Here's how the part is built. I have some questions about the finished solid (model axes, mm). A direction names the side the tool comes from. Give positions to 0.01 mm unless a question says otherwise; leave off trailing zeros. Order: outer loops, then holes, each group sorted by start corner. A loop starts at its lowest first (then second) coordinate and runs counter-clockwise, first axis right, second up. Notation, with made-up numbers: (73, 72) -> (106, 72) arc R21 cw to (106, 87) -> close; hole circle Ø6 at (-5, 22.25). An arc over 180 degrees is marked (long way). Write each question's results on one line, items separated by ' | '. Start each with the question number.
Q1. Imagine slicing it at B-B, the plane z = -34. State how many separate pieces and enclosed holes the cut face has, then the cut area to 3 significant figures.
Q2. I need wall thicknesses on line 1 along X through (y, z) = (13, -24); line 2 along Z through (x, y) = (69, 6.75); line 3 along Z through (x, y) = (31, 14). Which ranges of each line are inside material? Lowest first, please. Write a range as [from, to].
Q3. Thinking about a two-plate mould opening in Y: for faces 1 (the face through (95.504, 13, -17)), 2 (the face through (22, 25.375, -19)), 3 (the face through (81.08, 12.74, -14.7)), which applies, pulls with the +Y half, pulls with the -Y half, needs draft (parallel to the pull), parting line crosses it, or undercut?
Q4. I'm going to push flat-ended pins straight in: pin 1 (4 mm diameter, centred on x = 49.784, z = 0, fed in from -Y); pin 2 (13 mm diameter, centred on x = 69.85, y = 12.7, fed in from -Z); pin 3 (1 mm diameter, centred on x = 20.5, z = -9, fed in from -Y); pin 4 (1 mm diameter, centred on x = 16.5, y = 7.5, fed in from +Z). Where does each tip first touch, or does it pass through?
Q5. Imagine slicing it at C-C, the plane y = 2.5. Please give me the cut outline in (x, z), then the cut area to 3 significant figures.
Q6. For faces 4 (the face through (70, 0, -17)), 5 (the face through (75.156, 14.371, -25.858)), 6 (the face through (65.25, 14.37, -8.33)), which set-ups out of +Z, -Z, +X, -X, +Y, -Y let a thin tool reach every point of the face, with its end or its side?
```python
from build123d import *

# Parameters (mm, degrees)
BOSS_EXTRUDE1_DEPTH = 25.4
SKETCH2_W           = 44.704
SKETCH2_H           = 0.0254
CUT_EXTRUDE1_DEPTH  = 107.377492525
SKETCH3_R           = 2.286
CUT_EXTRUDE2_DEPTH  = 107.377492525


# Read off the part's stored shape, not the designer's step: 1/4 NPT Tapped Hole1
with BuildPart() as part:
    # Sketch1 → Boss-Extrude1 (new body)
    with BuildSketch(Plane(origin=(0, 0, 0), x_dir=(1, 0, 0), z_dir=(0, 1, 0))):
        Polygon((44.704, -5.08), (95.504, -5.08), (95.504, 39.37), (0, 39.37), (0, 0), (44.704, 0), align=None)
    extrude(amount=BOSS_EXTRUDE1_DEPTH)

    # Sketch2 → Cut-Extrude1 (cut, through all)
    with BuildSketch(Plane.XY):
        with Locations((22.352, 25.3873)):
            Rectangle(SKETCH2_W, SKETCH2_H)
        with Locations((22.352, 0.0127)):
            Rectangle(SKETCH2_W, SKETCH2_H)
    extrude(amount=-CUT_EXTRUDE1_DEPTH, mode=Mode.SUBTRACT)

    # Sketch3 → Cut-Extrude2 (cut, through all)
    with BuildSketch(Plane(origin=(0, 25.4, 0), x_dir=(1, 0, 0), z_dir=(0, 1, 0))):
        with Locations(Location((49.784, 0, 0), (0, 0, 270))):
            Circle(SKETCH3_R)
        with Locations(Location((84.328, 34.544, 0), (0, 0, 270))):
            Circle(SKETCH3_R)
    extrude(amount=-CUT_EXTRUDE2_DEPTH, mode=Mode.SUBTRACT)

    # 1/4 NPT Tapped Hole1 outline → 1/4 NPT Tapped Hole1 (revolve, cut)
    with BuildSketch(Plane(origin=(69.85, 12.7, 0), x_dir=(1, 0, 0), z_dir=(0, -1, 0))):
        Polygon((5.5626, -22.352), (0, -19.009652721), (0, -39.37), (6.8545837, -39.37), (6.557984794, -29.464), (5.5626, -29.464), align=None)
    revolve(axis=Axis((69.85, 12.7, 0), (0, 0, 1)), mode=Mode.SUBTRACT)

    # 1_4 NPT Tapped Hole1 2 outline → 1_4 NPT Tapped Hole1 2 (revolve, cut)
    with BuildSketch(Plane(origin=(82.042, 12.7, 0), x_dir=(1, 0, 0), z_dir=(0, -1, 0))):
        Polygon((0, 5.08), (0, -15.280347279), (5.5626, -11.938), (5.5626, -4.826), (6.557984794, -4.826), (6.8545837, 5.08), align=None)
    revolve(axis=Axis((82.042, 12.7, 0), (0, 0, 1)), mode=Mode.SUBTRACT)

    # 1_4 NPT Tapped Hole1 3 outline → 1_4 NPT Tapped Hole1 3 (revolve, cut)
    with BuildSketch(Plane(origin=(59.944, 12.7, 0), x_dir=(1, 0, 0), z_dir=(0, -1, 0))):
        Polygon((6.8545837, 5.08), (0, 5.08), (0, -15.280347279), (5.5626, -11.938), (5.5626, -4.826), (6.557984794, -4.826), align=None)
    revolve(axis=Axis((59.944, 12.7, 0), (0, 0, 1)), mode=Mode.SUBTRACT)


solid = part.part
```
Geometry check:
1) separate pieces: 2 | enclosed holes: 1 | area: 2,170 mm²
2) line 1: [0, 64.3], [75.4, 95.5] | line 2: [-29.46, 5.08] | line 3: [-39.37, 0]
3) face 1: needs draft | face 2: pulls with the +Y half | face 3: undercut
4) pin 1: through | pin 2: z = -29.46 | pin 3: y = 0.03 | pin 4: z = 0
5) outline: (0, -39.37) -> (95.5, -39.37) -> (95.5, 5.08) -> (44.7, 5.08) -> (44.7, 0) -> (0, 0) -> close; hole circle Ø4.57 at (49.78, 0); hole circle Ø4.57 at (84.33, -34.54) | area: 3,990 mm²
6) face 4: +Z, -Z, +X, -X, -Y | face 5: -Z | face 6: +Z
